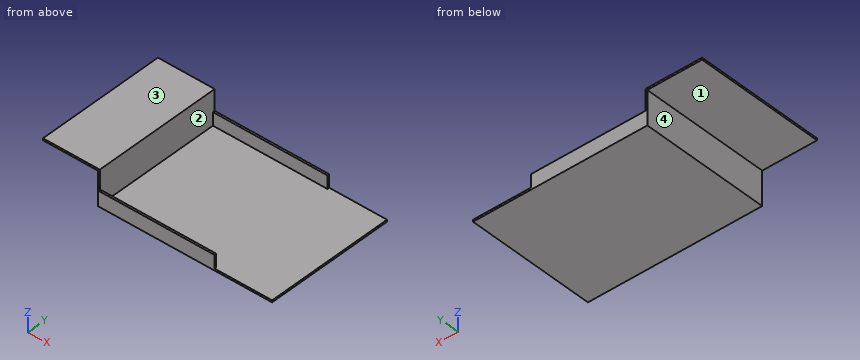
from build123d import *

# Parameters (mm, degrees)
SKETCH1_W           = 175
SKETCH1_H           = 130
BOSS_EXTRUDE1_DEPTH = 2
SKETCH2_W           = 2
SKETCH2_H           = 130
BOSS_EXTRUDE2_DEPTH = 34
SKETCH3_W           = 2
SKETCH3_H           = 130
BOSS_EXTRUDE4_DEPTH = 55
SKETCH5_W           = 115
SKETCH5_H           = 2
BOSS_EXTRUDE5_DEPTH = 13


with BuildPart() as part:
    # Sketch1 → Boss-Extrude1 (new body)
    with BuildSketch(Plane.XY):
        with Locations((87.5, 65)):
            Rectangle(SKETCH1_W, SKETCH1_H)
    extrude(amount=BOSS_EXTRUDE1_DEPTH)

    # Sketch2 → Boss-Extrude2 (add)
    with BuildSketch(Plane.XY.offset(2)):
        with Locations((1, 65)):
            Rectangle(SKETCH2_W, SKETCH2_H)
    extrude(amount=BOSS_EXTRUDE2_DEPTH)

    # Sketch3 → Boss-Extrude4 (add)
    with BuildSketch(Plane.ZY):
        with Locations((35, 65)):
            Rectangle(SKETCH3_W, SKETCH3_H)
    extrude(amount=BOSS_EXTRUDE4_DEPTH)

    # Sketch5 → Boss-Extrude5 (add)
    with BuildSketch(Plane.XY.offset(2)):
        with Locations((59.5, 1)):
            Rectangle(SKETCH5_W, SKETCH5_H)
        with Locations((59.5, 129)):
            Rectangle(SKETCH5_W, SKETCH5_H)
    extrude(amount=BOSS_EXTRUDE5_DEPTH)


solid = part.part
Geometry check sheet. Reference: the model listing, model coordinates, mm. Face numbers are marked on the shaded views. A direction names the side the tool comes from. Give positions to 0.01 mm unless a question says otherwise; leave off trailing zeros. Loops run counter-clockwise (first coordinate to the right, second up) from the corner with the lowest first, then second, coordinate; pieces in that order, holes last. Notation, with made-up numbers: (21.5, -3.75) -> (48.5, -3.75) arc R32 cw to (48.5, 25.25) -> close; hole circle Ø2 at (-14.75, 50.5). An arc over 180 degrees is marked (long way). Answer in a Markdown table with one row per item. Add a question column.
1) Cross-section at B-B on z = 10. Record the boundary of the cut face in (x, y).
2) Gauge pin test, flat ends, axial feed: P1, Ø1.6, axis at x = 33, y = 1.5, coming from the +Z side; P2, Ø10, axis at x = 145, y = 112.5, coming from the +Z side; P3, Ø1, axis at y = 89, z = 21.5, coming from the +X side. Record the tip position at first contact, or that the pin passes through.
3) Set-up check for the marked faces 3 and 4: record each of +Z, -Z, +X, -X, +Y, -Y from which the full face is reachable in a straight line by a thin tool's end or side.
4) Cross-section at D-D on x = 150. Record the boundary of the cut face in (y, z), and give its area (3 significant figures).
5) Material ranges on probe 1 along Y at (x, z) = (22, 4.5); probe 2 along X at (y, z) = (95, 20), recorded low to high. Write a range as from..to.
6) Cross-section at A-A on x = 9.5. Record the boundary of the cut face in (y, z).
7) Cross-section at C-C on z = 24.5. Record the boundary of the cut face in (x, y).
8) Draft check along Y on the marked faces 1 and 2. Enter one of: pulls with the +Y half, pulls with the -Y half, needs draft (parallel to the pull), parting line crosses it, or undercut.
Outcome:
| question | item | result |
|---|---|---|
| 1 | outline | (0, 0) -> (117, 0) -> (117, 2) -> (2, 2) -> (2, 128) -> (117, 128) -> (117, 130) -> (0, 130) -> close |
| 2 | P1 | stops at z = 15 |
| 2 | P2 | stops at z = 2 |
| 2 | P3 | stops at x = 2 |
| 3 | face 3 | +Z, +X, -X, +Y, -Y |
| 3 | face 4 | -Z, -X, +Y, -Y |
| 4 | outline | (0, 0) -> (130, 0) -> (130, 2) -> (0, 2) -> close |
| 4 | area | 260 mm^2 |
| 5 | probe 1 | y = 0..2, 128..130 |
| 5 | probe 2 | x = 0..2 |
| 6 | outline | (0, 0) -> (130, 0) -> (130, 15) -> (128, 15) -> (128, 2) -> (2, 2) -> (2, 15) -> (0, 15) -> close |
| 7 | outline | (0, 0) -> (2, 0) -> (2, 130) -> (0, 130) -> close |
| 8 | face 1 | needs draft |
| 8 | face 2 | undercut |
